For this review, use the dimensioned drawing (mm, ordinates from the lowest corner) and the shaded views. Round coordinates to 2 decimals unless told otherwise and drop trailing zeros. Loops run counter-clockwise (first coordinate to the right, second up) from the corner with the lowest first, then second, coordinate; pieces in that order, holes last. Notation, with made-up numbers: M 16,41 L 46,41 A34 ccw 46,77 Z; hole C 3.25,84 d3. An arc over 180 degrees is marked long. Use a Markdown table: item, result. Add a question column.
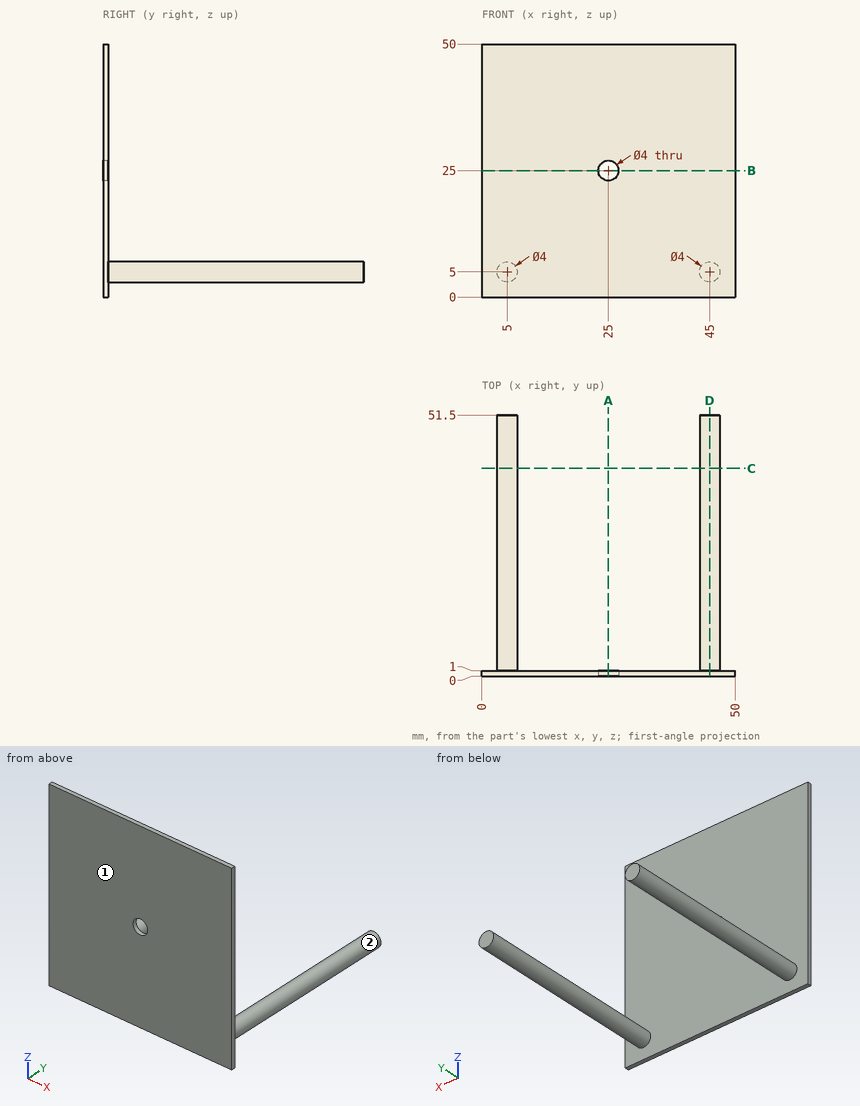
(1) Consider section A-A, the plane x = 25. Give the boundary of the cut face in (y, z).
(2) Consider section B-B, the plane z = 25. Give the boundary of the cut face in (x, y).
(3) Draft analysis for pull direction X (two halves, no side actions). For the marked faces 1 and 2, state which applies: released by +X, released by -X, zero draft, split by the parting line, or undercut.
(4) Consider section C-C, the plane y = 41. Give the boundary of the cut face in (x, z).
(5) Consider section D-D, the plane x = 45. Give the boundary of the cut face in (y, z), then the cut area to 3 significant figures.
(6) Insertion check: pin 1 Ø5 at (x, z) = (25, 25) entering from -Y; pin 2 Ø2 at (x, z) = (34.5, 21) entering from +Y; pin 3 Ø10 at (y, z) = (12.5, 11.5) entering from -X. Each pin has a flat end and moves straight along its axis. Give the tip position at first contact, or say it passes through.
(7) To check wall thickness, follow probe 1 along X at (y, z) = (0.65, 25); probe 2 along Y at (x, z) = (24.5, 47); probe 3 along Z at (x, y) = (4, 23.5). State the ranges of each line that lie inside material, in increasing order.
Found:
| question | item | result |
|---|---|---|
| 1 | outline | M 0,0 L 1,0 L 1,23 L 0,23 Z; M 0,27 L 1,27 L 1,50 L 0,50 Z |
| 2 | outline | M 0,0 L 23,0 L 23,1 L 0,1 Z; M 27,0 L 50,0 L 50,1 L 27,1 Z |
| 3 | face 1 | zero draft |
| 3 | face 2 | undercut |
| 4 | outline | C 5,5 d4; C 45,5 d4 |
| 5 | outline | M 0,0 L 1,0 L 1,3 L 51.5,3 L 51.5,7 L 1,7 L 1,50 L 0,50 Z |
| 5 | area | 252 mm^2 |
| 6 | pin 1 | stops at y = 0 |
| 6 | pin 2 | stops at y = 1 |
| 6 | pin 3 | stops at x = 3.68 |
| 7 | probe 1 | x = 0 to 23, 27 to 50 |
| 7 | probe 2 | y = 0 to 1 |
| 7 | probe 3 | z = 3.27 to 6.73 |
